```python
from build123d import *

# Parameters (mm, degrees)
F0_W     = 9
F0_H     = 32
F1_DEPTH = 1
F2_W     = 6.2
F2_H     = 6.3
F3_DEPTH = 2.6
F4_R     = 1.5
F5_DEPTH = 0.3
F5_TAPER = 10
F6_R     = 1.5


with BuildPart() as f1:
    # F0 (on Top) → F1 (new body)
    with BuildSketch(Plane.XY):
        Rectangle(F0_W, F0_H)
    extrude(amount=F1_DEPTH)

    # F2 (on face) → F3 (join)
    with BuildSketch(Plane.XY.offset(1)):
        with Locations((0, -8.85)):
            Rectangle(F2_W, F2_H)
    extrude(amount=F3_DEPTH)

    # F4 (on face) → F5 (join)
    with BuildSketch(Plane.XY.offset(3.6)):
        with Locations((0, -8.9)):
            Circle(F4_R)
    extrude(amount=F5_DEPTH, taper=F5_TAPER)

    # F6
    f6_edges = [f1.edges().sort_by_distance(p)[0] for p in [
        (4.5, -16, 0.5),
        (-4.5, -16, 0.5),
        (4.5, 16, 0.5),
        (-4.5, 16, 0.5),
    ]]
    fillet(f6_edges, radius=F6_R)


solid = f1.part
```
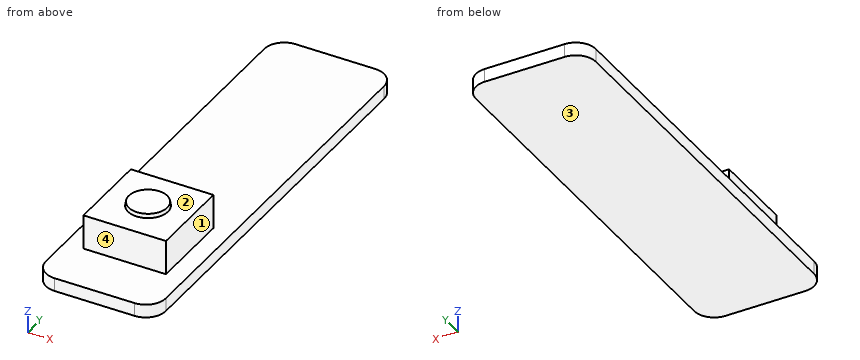
Work out the finished part from the listing and answer in its coordinate system (mm). Face numbers are marked on the shaded views. A direction names the side the tool comes from. Give positions to 0.01 mm unless a question says otherwise; leave off trailing zeros. Loops run counter-clockwise (first coordinate to the right, second up) from the corner with the lowest first, then second, coordinate; pieces in that order, holes last. Notation, with made-up numbers: M 20,72.5 L 25,72.5 A25 ccw 25,94.5 Z; hole C -12,53.5 d1. An arc over 180 degrees is marked long. One line per item, written item: value. Start each with the question number.
1. Which of the six approach directions +Z, -Z, +X, -X, +Y, -Y give full straight-line access (tool end or side, diameter ignored) to the marked faces 1, 2, 3 and 4?
2. Find section D-D (y = 8.5). Give the vertices of the cut face in (x, z).
3. Each of these flat-tipped pins is pushed along its axis until it touches: P1, Ø0.8, axis at y = -8.5, z = 2, coming from the -X side; P2, Ø1.5, axis at x = 2, y = -6, coming from the +Z side; P3, Ø0.8, axis at x = 0.5, z = 2.5, coming from the +Y side. Where does it stop, or does it pass through?
4. Find the intervals of material crossed by probe 1 along Z at (x, y) = (-2, 14); probe 2 along Y at (x, z) = (-0.5, 2.45); probe 3 along X at (y, z) = (-10, 2.2), in increasing order.
5. Find section A-A (x = 0). Give the vertices of the cut face in (y, z), and give its area (3 significant figures).
6. Find section B-B (y = -8.9). Give the vertices of the cut face in (x, z).
7. Find section C-C (z = 1.75). Give the vertices of the cut face in (x, y).
Reported:
1. face 1: +Z, +X, +Y, -Y
1. face 2: +Z
1. face 3: -Z, +X, -X, +Y, -Y
1. face 4: +Z, +X, -X, -Y
2. outline: M -4.5,0 L 4.5,0 L 4.5,1 L -4.5,1 Z
3. P1: stops at x = -3.1
3. P2: stops at z = 3.6
3. P3: stops at y = -5.7
4. probe 1: z = 0 to 1
4. probe 2: y = -12 to -5.7
4. probe 3: x = -3.1 to 3.1
5. outline: M -16,0 L 16,0 L 16,1 L -5.7,1 L -5.7,3.6 L -7.4,3.6 L -7.45,3.9 L -10.35,3.9 L -10.4,3.6 L -12,3.6 L -12,1 L -16,1 Z
5. area: 49.3 mm²
6. outline: M -4.5,0 L 4.5,0 L 4.5,1 L 3.1,1 L 3.1,3.6 L 1.5,3.6 L 1.45,3.9 L -1.45,3.9 L -1.5,3.6 L -3.1,3.6 L -3.1,1 L -4.5,1 Z
7. outline: M -3.1,-12 L 3.1,-12 L 3.1,-5.7 L -3.1,-5.7 Z
